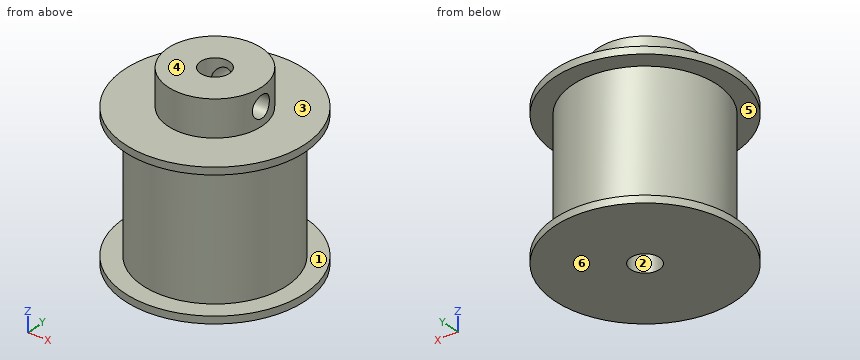
Autodesk Inventor part; units mm, degrees
ref_plane "Work Plane1" through (0, 0, 10) normal (0, 0, -1) x (-1, 0, 0)
ref_plane "YZ Plane" through (0, 0, 0) normal (1, 0, 0) x (0, 1, 0)
ref_plane "XZ Plane" through (0, 0, 0) normal (0, 1, 0) x (-1, 0, 0)
sketch "Sketch1" plane through (0, 0, 0) normal (0, 0, 1) x (1, 0, 0)
  circle A0 centre (0, 0) radius 12.5
  circle A1 centre (0, 0) radius 2
  dimension "d0" = 25
  dimension "d1" = 4
extrude "Extrusion1" add sketch "Sketch1" along normal blind 20
sketch "Sketch2" plane through (0, 0, 20) normal (0, 0, 1) x (1, 0, 0)
  circle A0 centre (0, 0) radius 2
  circle A1 centre (0, 0) radius 6.5
  dimension "d4" = 13
extrude "Extrusion2" add sketch "Sketch2" along normal blind 5
ref_plane "Work Plane1" through (0, 0, 10) normal (0, 0, -1) x (-1, 0, 0)
sketch "Sketch3" plane through (0, 0, 10) normal (0, 0, -1) x (-1, 0, 0)
  circle A0 centre (0, 0) radius 10
  circle A1 centre (0, 0) radius 12.5
  dimension "d7" = 20
extrude "Extrusion3" cut sketch "Sketch3" along normal mid plane 18
sketch "Sketch6" plane through (0, 0, 0) normal (0, 1, 0) x (-1, 0, 0)
  line L0 (6.5, 25) -> (-6.5, 25)
  line L1 (-6.5, 20) -> (6.5, 20)
  line L2 (-2, 25) -> (2, 25)
  line L3 (-2, 25) -> (2, 25)
  line L4 (2, 0) -> (-2, 0)
  circle A0 centre (0, 22.5) radius 1.5
  line L5 (6.5, 20) -> (6.5, 25)
  line L6 (-6.5, 20) -> (-6.5, 25)
  point P0 (0, 0)
  point P1 (0, 20)
  point P2 (6.5, 22.5)
  dimension "d36" = 3
extrude "Extrusion4" cut sketch "Sketch6" along normal through all contours A0
sketch "Sketch7" plane through (0, 0, 0) normal (1, 0, 0) x (0, 1, 0)
  line L0 (-2, 25) -> (2, 25)
  line L1 (6.5, 20) -> (6.5, 25)
  circle A0 centre (0, 22.5) radius 1.5
  point P0 (0, 0)
  point P1 (0, 25)
  point P2 (6.5, 22.5)
  dimension "d39" = 3
extrude "Extrusion5" cut sketch "Sketch7" along normal through all
properties part number "Timing Belt - 8mm Bore 5mm Pitch 14 Teeth 15mm Wide" material "Aluminum 6061"
Geometry: final body of the model. Coordinates: model frame, mm. Face numbers are marked on the shaded views. A direction names the side the tool comes from. Round coordinates to 2 decimals unless told otherwise and drop trailing zeros. Order: outer loops, then holes, each group sorted by start corner. A loop starts at its lowest first (then second) coordinate and runs counter-clockwise, first axis right, second up. Notation, with made-up numbers: (49, 77.25) -> (78, 77.25) arc R14 ccw to (78, 86.25) -> close; hole circle Ø1 at (56.5, 63.25). An arc over 180 degrees is marked (long way). Put each result on its own line as item: value. Start each with the question number.
Q1. Reachability of the marked faces 1, 2 and 3 from +Z, -Z, +X, -X, +Y, -Y: full face, straight path, thin tool, end or side. Return the list, or none.
Q2. Section C-C on z = 22.5. Return the cut outline in (x, y).
Q3. Line query: probe 1 along Z at (x, y) = (-6.75, -10.25); probe 2 along Z at (x, y) = (4.3, 0); probe 3 along Z at (x, y) = (-8, 1.5). Output: solid intervals per line, ascending.
Q4. Pull-direction query (Z, two-part tool) for the marked faces 4, 5 and 6; classes: +Z half, -Z half, draft (parallel to the pull), parting line (faces both ways), or undercut.
Q5. Section A-A on x = 0. Return the cut outline in (y, z).
Q6. First-contact query: pin 1 (1.5 mm diameter, centred on y = -4, z = 4, fed in from +X); pin 2 (4 mm diameter, centred on x = -5, y = 9.5, fed in from +Z); pin 3 (3 mm diameter, centred on y = 6.5, z = 13.5, fed in from +X). Flat tips, straight axial feed; report the tip coordinate or a pass-through.
Q7. Section D-D on x = -5. Return the cut outline in (y, z), and give its area (3 significant figures).
Ans:
1. face 1: none
1. face 2: +Z, -Z
1. face 3: +Z
2. outline: (-1.5, 1.32) -> (-1.5, 6.32) arc R6.5 ccw (long way) to (6.32, -1.5) -> (1.32, -1.5) arc R2 cw to start; (1.5, 1.5) -> (6.32, 1.5) arc R6.5 ccw to (1.5, 6.32) -> close
3. probe 1: z = 0 to 1, 19 to 20
3. probe 2: z = 0 to 21, 24 to 25
3. probe 3: z = 0 to 20
4. face 4: +Z half
4. face 5: undercut
4. face 6: -Z half
5. outline: (-12.5, 0) -> (-2, 0) -> (-2, 25) -> (-6.5, 25) -> (-6.5, 20) -> (-12.5, 20) -> (-12.5, 19) -> (-10, 19) -> (-10, 1) -> (-12.5, 1) -> close; (2, 0) -> (12.5, 0) -> (12.5, 1) -> (10, 1) -> (10, 19) -> (12.5, 19) -> (12.5, 20) -> (6.5, 20) -> (6.5, 21) -> (2, 21) -> close; (2, 24) -> (6.5, 24) -> (6.5, 25) -> (2, 25) -> close
6. pin 1: stops at x = 9.46
6. pin 2: stops at z = 20
6. pin 3: stops at x = 8.66
7. outline: (-11.46, 0) -> (11.46, 0) -> (11.46, 1) -> (8.66, 1) -> (8.66, 19) -> (11.46, 19) -> (11.46, 20) -> (4.15, 20) -> (4.15, 25) -> (-4.15, 25) -> (-4.15, 20) -> (-11.46, 20) -> (-11.46, 19) -> (-8.66, 19) -> (-8.66, 1) -> (-11.46, 1) -> close
7. area: 399 mm2
